Geometry check sheet. Reference: the model listing, model coordinates, mm. Face numbers are marked on the shaded views. A direction names the side the tool comes from. Coordinates: 2 decimals unless noted, no trailing zeros. Write each loop counter-clockwise with the first axis right and the second up, starting at its lowest first coordinate (ties: lowest second). Pieces come first, ordered by that corner, then holes.
from build123d import *

# Parameters (mm, degrees)
SKETCH_1_W                          = 440
SKETCH_1_H                          = 1392
EXTRUDE_1_DEPTH                     = 1.5
SKETCH_5_W                          = 22
SKETCH_5_H                          = 105
CUT_EXTRUDE_4_DEPTH                 = 5
SKETCH_2_R                          = 3.3
CUT_EXTRUDE_1813_DEPTH              = 10
CUT_EXTRUDE_2195_DEPTH              = 10
SKETCH_8_R                          = 5.5
CUT_EXTRUDE_3659_DEPTH              = 1.5
CUT_EXTRUDE_4343_DEPTH              = 730.944004702
CUT_EXTRUDE_4343_DEPTH_BACK         = 730.944004702
SKETCH_21_W                         = 72
SKETCH_21_H                         = 8
SKETCH_21_W_2                       = 50
SKETCH_21_H_2                       = 5
SM_EDGE_FLANGE_2_STRIP_W            = 10
SM_EDGE_FLANGE_2_STRIP_H            = 1.5
SM_EDGE_FLANGE_2_STRIP_CUT_DEPTH    = 929
SM_EDGE_FLANGE_2_RELIEF_W           = 10.75
SM_EDGE_FLANGE_2_RELIEF_H           = 0.75
SM_EDGE_FLANGE_2_RELIEF_CUT_DEPTH   = 1.5
SM_EDGE_FLANGE_2_STRIP_2_W          = 10
SM_EDGE_FLANGE_2_STRIP_2_H          = 1.5
SM_EDGE_FLANGE_2_STRIP_CUT_2_DEPTH  = 929
SM_EDGE_FLANGE_2_RELIEF_2_W         = 10.75
SM_EDGE_FLANGE_2_RELIEF_2_H         = 0.75
SM_EDGE_FLANGE_2_RELIEF_CUT_2_DEPTH = 1.5
SM_EDGE_FLANGE_2_DEPTH              = 929
SM_EDGE_FLANGE_2_BEND_DEPTH         = 929
SKETCH_32_W                         = 2.75
SKETCH_32_H                         = 349.25
CUT_EXTRUDE_7725_DEPTH              = 1.5
FILLET_5_R                          = 3


# Sheet-metal steps are written as plain solids
with BuildPart() as part:
    # Эскиз1 → Бобышка-Вытянуть1 (new body)
    with BuildSketch(Plane.XY):
        Rectangle(SKETCH_1_W, SKETCH_1_H)
    extrude(amount=EXTRUDE_1_DEPTH)

    # Эскиз5 → Вырез-Вытянуть4 (cut)
    with BuildSketch(Plane.XY.offset(1.5)):
        with Locations((-209, 643.5)):
            Rectangle(SKETCH_5_W, SKETCH_5_H)
        with Locations((209, 643.5)):
            Rectangle(SKETCH_5_W, SKETCH_5_H)
    extrude(amount=-CUT_EXTRUDE_4_DEPTH, mode=Mode.SUBTRACT)

    # Эскиз2 → Cut-Extrude 1813 (cut)
    with BuildSketch(Plane.XY.offset(1.5)):
        with Locations((-150, 50)):
            Circle(SKETCH_2_R)
        with Locations(Location((-150, -50, 0), (0, 0, 180))):
            Circle(SKETCH_2_R)
        with Locations((150, -50)):
            Circle(SKETCH_2_R)
        with Locations(Location((150, 50, 0), (0, 0, 180))):
            Circle(SKETCH_2_R)
    extrude(amount=-CUT_EXTRUDE_1813_DEPTH, mode=Mode.SUBTRACT)

    # Sketch 3 → Cut-Extrude 2195 (cut)
    with BuildSketch(Plane.XY.offset(1.5)):
        with BuildLine():
            Line((-185, 611), (-185, 676))
            ThreePointArc((-185, 676), (-175, 686), (-165, 676))
            Line((-165, 676), (-165, 611))
            ThreePointArc((-165, 611), (-175, 601), (-185, 611))
        make_face()
        with BuildLine():
            Line((-185, 516), (-185, 581))
            ThreePointArc((-185, 581), (-175, 591), (-165, 581))
            Line((-165, 581), (-165, 516))
            ThreePointArc((-165, 516), (-175, 506), (-185, 516))
        make_face()
        with BuildLine():
            Line((165, 516), (165, 581))
            ThreePointArc((165, 581), (175, 591), (185, 581))
            Line((185, 581), (185, 516))
            ThreePointArc((185, 516), (175, 506), (165, 516))
        make_face()
        with BuildLine():
            Line((165, 611), (165, 676))
            ThreePointArc((165, 676), (175, 686), (185, 676))
            Line((185, 676), (185, 611))
            ThreePointArc((185, 611), (175, 601), (165, 611))
        make_face()
    extrude(amount=-CUT_EXTRUDE_2195_DEPTH, mode=Mode.SUBTRACT)

    # Эскиз8 → Cut-Extrude 3659 (cut)
    with BuildSketch(Plane.XY.offset(1.5)):
        with Locations((183, -646)):
            Circle(SKETCH_8_R)
        with Locations((-183, -646)):
            Circle(SKETCH_8_R)
        with Locations((183, 473)):
            Circle(SKETCH_8_R)
        with Locations((-183, 473)):
            Circle(SKETCH_8_R)
    extrude(amount=-CUT_EXTRUDE_3659_DEPTH, mode=Mode.SUBTRACT)

    # Эскиз21 → Cut-Extrude 4343 (cut, two sides: drawn at the far end of the back side and taken through both)
    with BuildSketch(Plane.XY.offset(1.5).offset(-CUT_EXTRUDE_4343_DEPTH_BACK)):
        with Locations((-184, -692)):
            Rectangle(SKETCH_21_W, SKETCH_21_H)
        with Locations((-173, 693.5)):
            Rectangle(SKETCH_21_W_2, SKETCH_21_H_2)
        with Locations((184, -692)):
            Rectangle(SKETCH_21_W, SKETCH_21_H)
        with Locations((173, 693.5)):
            Rectangle(SKETCH_21_W_2, SKETCH_21_H_2)
    extrude(amount=CUT_EXTRUDE_4343_DEPTH + CUT_EXTRUDE_4343_DEPTH_BACK, mode=Mode.SUBTRACT)

    # Ребро-кромка2: sheet metal written as solids
    # Ребро-кромка2 strip (on a plane across the edge) → Ребро-кромка2 strip cut (cut)
    with BuildSketch(Plane(origin=(-220, -688, 0), x_dir=(1, 0, 0), z_dir=(0, 1, 0))):
        with Locations((-3, -0.75)):
            Rectangle(SM_EDGE_FLANGE_2_STRIP_W, SM_EDGE_FLANGE_2_STRIP_H)
    extrude(amount=SM_EDGE_FLANGE_2_STRIP_CUT_DEPTH, mode=Mode.SUBTRACT)

    # Ребро-кромка2 relief (on the sheet) → Ребро-кромка2 relief cut (cut)
    with BuildSketch(Plane(origin=(-218, -688, 0), x_dir=(1, 0, 0), z_dir=(0, 0, -1))):
        with Locations((-4.625, -929.375)):
            Rectangle(SM_EDGE_FLANGE_2_RELIEF_W, SM_EDGE_FLANGE_2_RELIEF_H)
    extrude(amount=-SM_EDGE_FLANGE_2_RELIEF_CUT_DEPTH, mode=Mode.SUBTRACT)

    # Ребро-кромка2 strip 2 (on a plane across the edge) → Ребро-кромка2 strip cut 2 (cut)
    with BuildSketch(Plane(origin=(220, 241, 0), x_dir=(-1, 0, 0), z_dir=(0, -1, 0))):
        with Locations((-3, -0.75)):
            Rectangle(SM_EDGE_FLANGE_2_STRIP_2_W, SM_EDGE_FLANGE_2_STRIP_2_H)
    extrude(amount=SM_EDGE_FLANGE_2_STRIP_CUT_2_DEPTH, mode=Mode.SUBTRACT)

    # Ребро-кромка2 relief 2 (on the sheet) → Ребро-кромка2 relief cut 2 (cut)
    with BuildSketch(Plane(origin=(218, 241, 0), x_dir=(-1, 0, 0), z_dir=(0, 0, -1))):
        with Locations((-4.625, 0.375)):
            Rectangle(SM_EDGE_FLANGE_2_RELIEF_2_W, SM_EDGE_FLANGE_2_RELIEF_2_H)
    extrude(amount=-SM_EDGE_FLANGE_2_RELIEF_CUT_2_DEPTH, mode=Mode.SUBTRACT)

    # Ребро-кромка2 section (on a plane across the edge) → Ребро-кромка2 (add)
    with BuildSketch(Plane(origin=(-220, -688, 0), x_dir=(1, 0, 0), z_dir=(0, 1, 0))):
        with BuildLine():
            Line((-1.5, 2), (-1.5, 13.5))
            Line((-1.5, 13.5), (0, 13.5))
            Line((0, 13.5), (0, 2))
            ThreePointArc((0, 2), (0.585786438, 0.585786438), (2, 0))
            Line((2, 0), (2, -1.5))
            ThreePointArc((2, -1.5), (-0.474873734, -0.474873734), (-1.5, 2))
        make_face()
    extrude(amount=SM_EDGE_FLANGE_2_DEPTH)

    # Ребро-кромка2 section 2 (on a plane across the edge) → Ребро-кромка2 bend (add)
    with BuildSketch(Plane(origin=(220, 241, 0), x_dir=(-1, 0, 0), z_dir=(0, -1, 0))):
        with BuildLine():
            Line((-1.5, 2), (-1.5, 13.5))
            Line((-1.5, 13.5), (0, 13.5))
            Line((0, 13.5), (0, 2))
            ThreePointArc((0, 2), (0.585786438, 0.585786438), (2, 0))
            Line((2, 0), (2, -1.5))
            ThreePointArc((2, -1.5), (-0.474873734, -0.474873734), (-1.5, 2))
        make_face()
    extrude(amount=SM_EDGE_FLANGE_2_BEND_DEPTH)

    # Эскиз32 → Cut-Extrude 7725 (cut)
    with BuildSketch(Plane.XY.offset(1.5)):
        with Locations((-218.625, 416.375)):
            Rectangle(SKETCH_32_W, SKETCH_32_H)
        with Locations((218.625, 416.375)):
            Rectangle(SKETCH_32_W, SKETCH_32_H)
    extrude(amount=-CUT_EXTRUDE_7725_DEPTH, mode=Mode.SUBTRACT)

    # Скругление5
    fillet_5_edges = [part.edges().sort_by_distance(p)[0] for p in [
        (-220.75, -688, -13.5),
        (-220.75, 241, -13.5),
        (220.75, 241, -13.5),
        (220.75, -688, -13.5),
        (-217.25, 591, 0.75),
        (217.25, 591, 0.75),
        (-148, 696, 0.75),
        (148, 696, 0.75),
        (198, 691, 0.75),
        (148, -696, 0.75),
        (-148, -696, 0.75),
        (-198, 691, 0.75),
    ]]
    fillet(fillet_5_edges, radius=FILLET_5_R)


solid = part.part
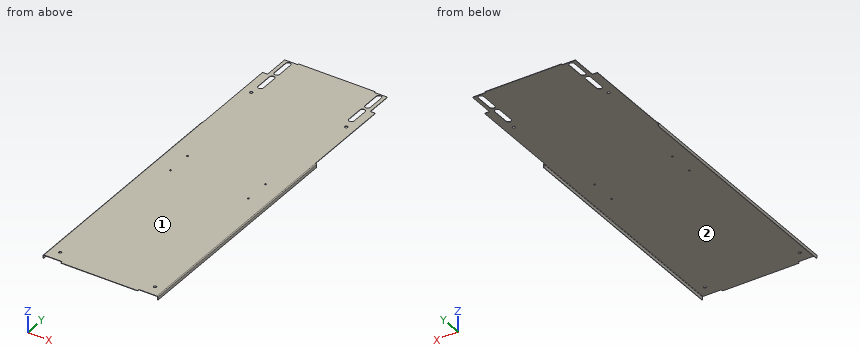
1. Sectioned sample at C-C, the plane x = 127. Record the boundary of the cut face in (y, z).
Computed values:
outline: (-696, 0) - (696, 0) - (696, 1.5) - (-696, 1.5) - close
2. Thickness scan on line 1 along Y through (x, z) = (150, 1.2); line 2 along X through (y, z) = (111.5, -7); line 3 along X through (y, z) = (-646, 1.15). Record the ranges inside material, lowest first.
Computed values:
line 1: y = -688 to -53.3, -46.7 to 46.7, 53.3 to 691
line 2: x = -221.5 to -220, 220 to 221.5
line 3: x = -219.53 to -188.5, -177.5 to 177.5, 188.5 to 219.53
3. Access from +Z, -Z, +X, -X, +Y, -Y to the whole of each face (thin tool, end or side, straight path). Record for the marked faces 1 and 2.
Computed values:
face 1: +Z, +X, -X, +Y, -Y
face 2: -Z, +Y, -Y
4. Sectioned sample at A-A, the plane z = -7.5. Record the boundary of the cut face in (x, y).
Computed values:
outline: (-221.5, -688) - (-220, -688) - (-220, 241) - (-221.5, 241) - close; (220, -688) - (221.5, -688) - (221.5, 241) - (220, 241) - close
5. Sectioned sample at D-D, the plane y = 455.5. Record the boundary of the cut face in (x, z), and give its area (3 significant figures).
Computed values:
outline: (-217.25, 0) - (217.25, 0) - (217.25, 1.5) - (-217.25, 1.5) - close
area: 652 mm2
6. Sectioned sample at B-B, the plane y = -599. Record the boundary of the cut face in (x, z).
Computed values:
outline: (-221.5, -13.5) - (-220, -13.5) - (-220, -2) arc R2 cw to (-218, 0) - (218, 0) arc R2 cw to (220, -2) - (220, -13.5) - (221.5, -13.5) - (221.5, -2) arc R3.5 ccw to (218, 1.5) - (-218, 1.5) arc R3.5 ccw to (-221.5, -2) - close
7. Gauge pin test, flat ends, axial feed: pin 1 Ø0.8 at (y, z) = (617, 1) entering from -X; pin 2 Ø1.2 at (y, z) = (642, 0.5) entering from +X; pin 3 Ø4 at (x, y) = (61.5, -322) entering from -Z. Record the tip position at first contact, or that the pin passes through.
Computed values:
pin 1: stops at x = -198
pin 2: stops at x = 198
pin 3: stops at z = 0
